The listing builds one solid part. Answer for the finished solid, in the listing's coordinates (mm). Give positions to 0.01 mm unless a question says otherwise; leave off trailing zeros. Write each loop counter-clockwise with the first axis right and the second up, starting at its lowest first coordinate (ties: lowest second). Pieces come first, ordered by that corner, then holes.
```python
from build123d import *

# Parameters (mm, degrees)
SKETCH1_R           = 6
BOSS_EXTRUDE1_DEPTH = 9.7


with BuildPart() as part:
    # Sketch1 → Boss-Extrude1 (new body)
    with BuildSketch(Plane(origin=(0, 0, 0), x_dir=(1, 0, 0), z_dir=(0, 1, 0))):
        Polygon((-10.910534447, 0), (-5.455267224, -9.4488), (5.455267224, -9.4488), (10.910534447, 0), (5.455267224, 9.4488), (-5.455267224, 9.4488), align=None)
        with Locations(Location((0, 0, 0), (0, 0, 270))):
            Circle(SKETCH1_R, mode=Mode.SUBTRACT)
    extrude(amount=BOSS_EXTRUDE1_DEPTH)

    # Sketch3 → Cut-Revolve3 (revolve, cut)
    with BuildSketch(Plane.XY, mode=Mode.PRIVATE) as cut_revolve3_sk:
        Polygon((-9.035534447, 9.7), (-10.910534447, 9.7), (-10.910534447, 7.825), align=None)
    revolve(cut_revolve3_sk.sketch.rotate(Axis((0, 0, 0), (0, 1, 0)), 270), axis=Axis((0, 0, 0), (0, 1, 0)), mode=Mode.SUBTRACT)

    # Sketch4 → Cut-Revolve4 (revolve, cut)
    with BuildSketch(Plane.XY, mode=Mode.PRIVATE) as cut_revolve4_sk:
        Polygon((-9.035534447, 0), (-10.910534447, 0), (-10.910534447, 1.875), align=None)
    revolve(cut_revolve4_sk.sketch.rotate(Axis((0, 0, 0), (0, 1, 0)), 270), axis=Axis((0, 0, 0), (0, 1, 0)), mode=Mode.SUBTRACT)


solid = part.part
```
Item 1: A cutting plane is placed at A-A, the plane x = 0. Give the vertices of the cut face in (y, z), plus the area to 3 significant figures.
Conclusion:
outline: (0, -9.04) - (0.41, -9.45) - (9.29, -9.45) - (9.7, -9.04) - (9.7, -6) - (0, -6) - close; (0, 6) - (9.7, 6) - (9.7, 9.04) - (9.29, 9.45) - (0.41, 9.45) - (0, 9.04) - close
area: 66.6 mm2
Item 2: Each of these flat-tipped pins is pushed along its axis until it touches: P1, Ø3, axis at x = -8.5, y = 8.5, coming from the +Z side; P2, Ø1, axis at y = 7, z = 2, coming from the +X side. Where does it stop, or does it pass through?
Conclusion:
P1: stops at z = 6.77
P2: stops at x = 10.04
Item 3: A cutting plane is placed at C-C, the plane y = 8.5. Give the vertices of the cut face in (x, z).
Conclusion:
outline: (-10.15, -1.32) - (-6.22, -8.13) arc R10.24 ccw to (-3.94, -9.45) - (3.94, -9.45) arc R10.24 ccw to (6.22, -8.13) - (10.15, -1.32) arc R10.24 ccw to (10.15, 1.32) - (6.22, 8.13) arc R10.24 ccw to (3.94, 9.45) - (-3.94, 9.45) arc R10.24 ccw to (-6.22, 8.13) - (-10.15, 1.32) arc R10.24 ccw to start; hole circle Ø12 at (0, 0)
Item 4: A cutting plane is placed at B-B, the plane y = 4.25. Give the vertices of the cut face in (x, z).
Conclusion:
outline: (-10.91, 0) - (-5.46, -9.45) - (5.46, -9.45) - (10.91, 0) - (5.46, 9.45) - (-5.46, 9.45) - close; hole circle Ø12 at (0, 0)
Item 5: Consider probe 1 along X at (y, z) = (6.5, -3.75); probe 2 along X at (y, z) = (5, 5.25); probe 3 along Z at (x, y) = (-3.75, 3.25). Determine where each line is inside the solid, lowest interval first.
Conclusion:
probe 1: x = -8.75 to -4.68, 4.68 to 8.75
probe 2: x = -7.88 to -2.9, 2.9 to 7.88
probe 3: z = -9.45 to -4.68, 4.68 to 9.45
Item 6: Determine the mould class of faces 1 (the face through (0, 5, 9.449)), 2 (the face through (1.802, 4.782, 5.723)), 3 (the face through (0, 5, -9.449)), 4 (the face through (6, 9.7, 2)) for opening direction Z: pulls with the +Z half, pulls with the -Z half, needs draft (parallel to the pull), parting line crosses it, or undercut.
Conclusion:
face 1: pulls with the +Z half
face 2: undercut
face 3: pulls with the -Z half
face 4: needs draft
